The listing builds one solid part. Answer for the finished solid, in the listing's coordinates (mm). Coordinates: 2 decimals unless noted, no trailing zeros. Loops run counter-clockwise (first coordinate to the right, second up) from the corner with the lowest first, then second, coordinate; pieces in that order, holes last. Notation, with made-up numbers: (-20, 16) - (-7, 16) arc R22 ccw to (-7, 36) - close; hole circle Ø10 at (-27.5, 28). An arc over 180 degrees is marked (long way). One line per question, with ' | ' between items.
from build123d import *

# Parameters (mm, degrees)
SKETCH1_W           = 242
SKETCH1_H           = 242
SKETCH1_W_2         = 105
SKETCH1_H_2         = 105
BOSS_EXTRUDE1_DEPTH = 3
CUT_EXTRUDE1_REACH  = 5
SKETCH2_R           = 7.5


with BuildPart() as part:
    # Sketch1 → Boss-Extrude1 (new body)
    with BuildSketch(Plane.XY):
        Rectangle(SKETCH1_W, SKETCH1_H)
        Rectangle(SKETCH1_W_2, SKETCH1_H_2, mode=Mode.SUBTRACT)
    extrude(amount=BOSS_EXTRUDE1_DEPTH)

    # Sketch2 → Cut-Extrude1 (cut, up to next)
    with BuildSketch(Plane.XY.offset(3), mode=Mode.PRIVATE) as cut_extrude1_sk1:
        with Locations((0, -91)):
            Circle(SKETCH2_R)
    cut_extrude1_tool1 = extrude(cut_extrude1_sk1.sketch, amount=-CUT_EXTRUDE1_REACH, mode=Mode.PRIVATE) & part.part
    add(cut_extrude1_tool1.solids().sort_by_distance((0, -91, 3))[0], mode=Mode.SUBTRACT)


solid = part.part
Item 1: Find section A-A, the plane x = -15. Write down the section's boundary in (y, z), plus the area to 3 significant figures.
Taken from the geometry:
outline: (-121, 0) - (-52.5, 0) - (-52.5, 3) - (-121, 3) - close; (52.5, 0) - (121, 0) - (121, 3) - (52.5, 3) - close | area: 411 mm2
Item 2: Find section B-B, the plane y = -91. Write down the section's boundary in (x, z).
Taken from the geometry:
outline: (-121, 0) - (-7.5, 0) - (-7.5, 3) - (-121, 3) - close; (7.5, 0) - (121, 0) - (121, 3) - (7.5, 3) - close
Item 3: Find the intervals of material crossed by line 1 (Y direction, x = 0, z = 1.15); line 2 (Y direction, x = 30, z = 2.6), in increasing order. Write a range as [from, to].
Taken from the geometry:
line 1: y = [-121, -98.5], [-83.5, -52.5], [52.5, 121] | line 2: y = [-121, -52.5], [52.5, 121]
Item 4: Find section C-C, the plane z = 1.15. Write down the section's boundary in (x, y), plus the area to 3 significant figures.
Taken from the geometry:
outline: (-121, -121) - (121, -121) - (121, 121) - (-121, 121) - close; hole (-52.5, -52.5) - (52.5, -52.5) - (52.5, 52.5) - (-52.5, 52.5) - close; hole circle Ø15 at (0, -91) | area: 47,400 mm2
Item 5: The mould has two halves that part along X. Classify faces 1 (the face through (3.461, -97.654, 1.521)), 2 (the face through (-55, 2, 0)): pulls with the +X half, pulls with the -X half, needs draft (parallel to the pull), parting line crosses it, or undercut.
Taken from the geometry:
face 1: undercut | face 2: needs draft
